Can you work these out from the model? Positions are in its coordinate system, mm. Face numbers are marked on the shaded views. Round coordinates to 2 decimals unless told otherwise and drop trailing zeros. Write each loop counter-clockwise with the first axis right and the second up, starting at its lowest first coordinate (ties: lowest second). Pieces come first, ordered by that corner, then holes.
Q1. I'm going to push flat-ended pins straight in: pin 1 Ø0.5 at (y, z) = (-24.5, 1) entering from +X; pin 2 Ø0.5 at (x, z) = (-0.5, 1) entering from +Y. Where does each tip first touch, or does it pass through?
Q2. We'd pull the mould along Z, two halves only. Please class the marked faces 1 and 2: +Z half, -Z half, draft (parallel to the pull), parting line (faces both ways), or undercut.
Q3. Please list where these lines run through material, in increasing order: line 1 along X through (y, z) = (-39.5, 1.3); line 2 along X through (y, z) = (-33, 0.95); line 3 along X through (y, z) = (-30.5, 0.3).
Q4. If we section it at C-C (x = 4.75): Please give me the cut outline in (y, z), plus the area to 3 significant figures.
Q5. If we section it at A-A (y = -40): Please give me the cut outline in (x, z), plus the area to 3 significant figures.
Q6. If we section it at B-B (z = 0.35): Please give me the cut outline in (x, y).
Q7. If we section it at D-D (y = -32.5): Please give me the cut outline in (x, z).
from build123d import *

# Parameters (mm, degrees)
BOSS_EXTRUDE1_DEPTH = 1.524


with BuildPart() as part:
    # Sketch1 → Boss-Extrude1 (new body)
    with BuildSketch(Plane.XY):
        with BuildLine():
            Line((-1.524, -34.676201819), (0, -34.676201819))
            Line((0, -34.676201819), (0, -20.584065252))
            ThreePointArc((0, -20.584065252), (4.472947003, -31.108201588), (7.416031026, -42.158222264))
            ThreePointArc((7.416031026, -42.158222264), (5.753516475, -40.272714916), (3.52711699, -39.105565432))
            ThreePointArc((3.52711699, -39.105565432), (5.686055365, -40.951036914), (7.416031026, -43.203583054))
            ThreePointArc((7.416031026, -43.203583054), (6.372439306, -49.781793421), (3.150525994, -55.611133859))
            ThreePointArc((3.150525994, -55.611133859), (-0.189129191, -59.717886603), (-4.674525994, -62.528568082))
            ThreePointArc((-4.674525994, -62.528568082), (-3.899739777, -59.06985097), (-4.674525994, -55.611133859))
            ThreePointArc((-4.674525994, -55.611133859), (-7.896439306, -49.781793421), (-8.940031026, -43.203583054))
            ThreePointArc((-8.940031026, -43.203583054), (-7.210055365, -40.951036914), (-5.05111699, -39.105565432))
            ThreePointArc((-5.05111699, -39.105565432), (-7.277516475, -40.272714916), (-8.940031026, -42.158222264))
            ThreePointArc((-8.940031026, -42.158222264), (-5.996947003, -31.108201588), (-1.524, -20.584065252))
            Line((-1.524, -20.584065252), (-1.524, -34.676201819))
        make_face()
    extrude(amount=BOSS_EXTRUDE1_DEPTH)


solid = part.part
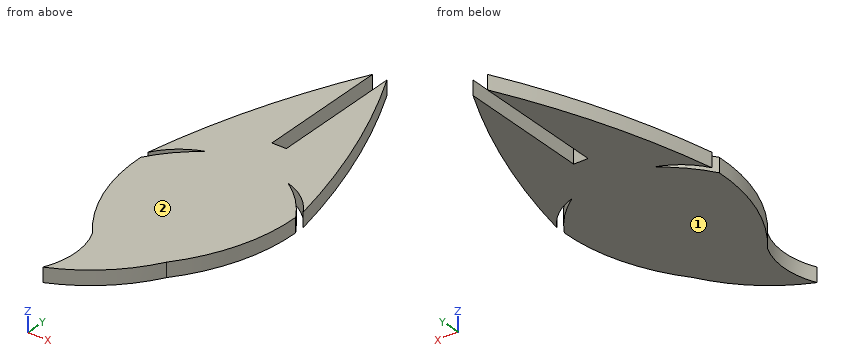
A:
1. pin 1: stops at x = 1.98
1. pin 2: stops at y = -34.68
2. face 1: -Z half
2. face 2: +Z half
3. line 1: x = -8.38 to -6.05, -5.59 to 4.07, 4.52 to 6.86
3. line 2: x = -6.62 to -1.52, 0 to 5.1
3. line 3: x = -5.79 to -1.52, 0 to 4.26
4. outline: (-53.3, 0) - (-40.05, 0) - (-40.05, 1.52) - (-53.3, 1.52) - close; (-39.62, 0) - (-31.93, 0) - (-31.93, 1.52) - (-39.62, 1.52) - close
4. area: 31.9 mm2
5. outline: (-8.5, 0) - (-6.91, 0) - (-6.91, 1.52) - (-8.5, 1.52) - close; (-6.21, 0) - (4.69, 0) - (4.69, 1.52) - (-6.21, 1.52) - close; (5.38, 0) - (6.97, 0) - (6.97, 1.52) - (5.38, 1.52) - close
5. area: 21.5 mm2
6. outline: (-8.94, -43.2) arc R19.26 ccw to (-4.67, -55.61) arc R8.11 cw to (-4.67, -62.53) arc R16.2 ccw to (3.15, -55.61) arc R19.26 ccw to (7.42, -43.2) arc R13.64 ccw to (3.53, -39.11) arc R6.92 cw to (7.42, -42.16) arc R80.83 ccw to (0, -20.58) - (0, -34.68) - (-1.52, -34.68) - (-1.52, -20.58) arc R80.83 ccw to (-8.94, -42.16) arc R6.92 cw to (-5.05, -39.11) arc R13.64 ccw to start
7. outline: (-6.46, 0) - (-1.52, 0) - (-1.52, 1.52) - (-6.46, 1.52) - close; (0, 0) - (4.94, 0) - (4.94, 1.52) - (0, 1.52) - close
